Verification items for this drawing (mm, ordinates from the low corner). A direction names the side the tool comes from. Round coordinates to 2 decimals unless told otherwise and drop trailing zeros. Loops run counter-clockwise (first coordinate to the right, second up) from the corner with the lowest first, then second, coordinate; pieces in that order, holes last. Notation, with made-up numbers: M -1,22.5 L 25,22.5 A34 cw 25,57.5 Z; hole C 88.5,18 d5. An arc over 180 degrees is marked long. Write item = value, one per line. Start each with the question number.
(1) Cross-section at B-B on y = 38. Record the boundary of the cut face in (x, z), plus the area to 3 significant figures.
(2) Cross-section at A-A on z = 6.5. Record the boundary of the cut face in (x, y), plus the area to 3 significant figures.
(3) Go/stop test with flat-tipped pins: P1, Ø2, axis at x = 18, z = 8.5, coming from the +Y side; P2, Ø3, axis at y = 26, z = 4.5, coming from the -X side. Record where each tip stops, or that it passes through.
(4) Set-up check for the marked faces 1 and 2: record each of +Z, -Z, +X, -X, +Y, -Y from which the full face is reachable in a straight line by a thin tool's end or side.
(5) Cross-section at C-C on x = 3.5. Record the boundary of the cut face in (y, z).
(6) Scan lines: L1, parallel to X at y = 29, z = 6.5; L2, parallel to Y at x = 11, z = 5.5. Record each from-to range of solid material in increasing order. Write a range as from..to.
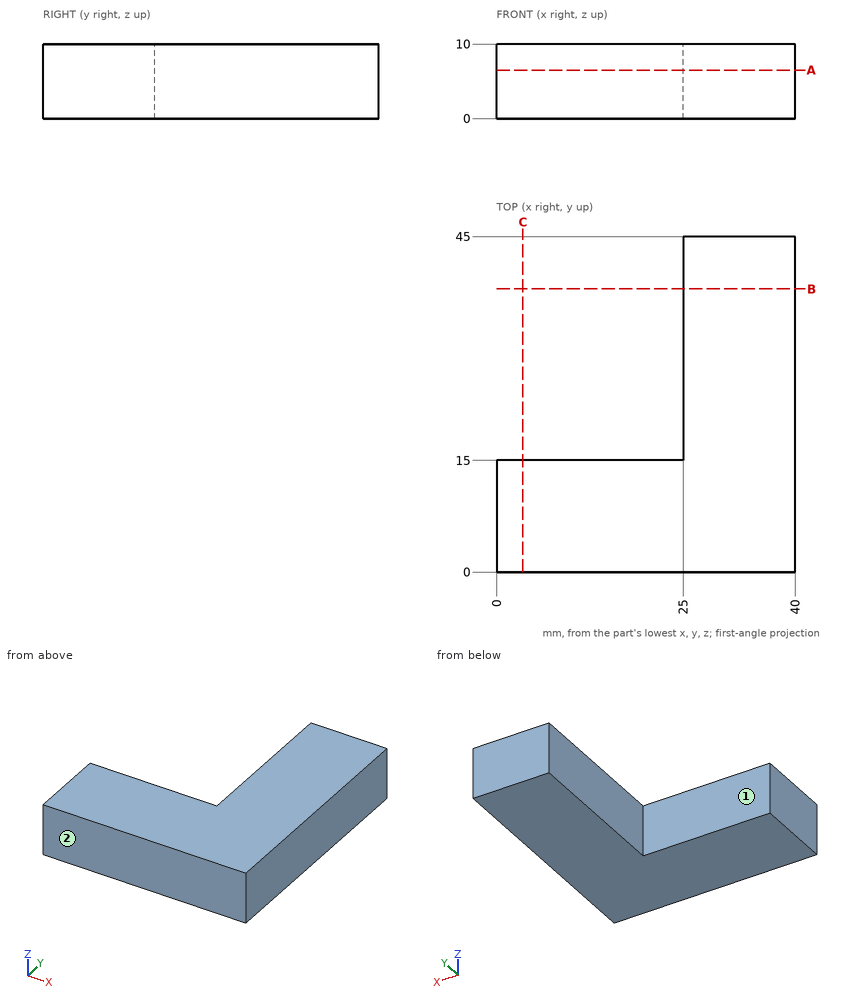
Result:
q1.outline = M 25,0 L 40,0 L 40,10 L 25,10 Z
q1.area = 150 mm^2
q2.outline = M 0,0 L 40,0 L 40,45 L 25,45 L 25,15 L 0,15 Z
q2.area = 1,050 mm^2
q3.P1 = 15
q3.P2 = 25
q4.face_1 = +Z, -Z, -X, +Y
q4.face_2 = +Z, -Z, +X, -X, -Y
q5.outline = M 0,0 L 15,0 L 15,10 L 0,10 Z
q6.L1 = 25..40
q6.L2 = 0..15
